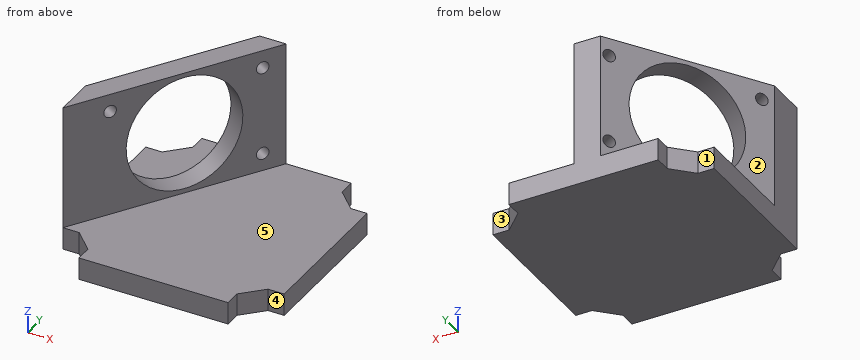
Autodesk Inventor part; units mm, degrees
ref_plane "Work Plane1" through (0, 0, 10) normal (0, 0, 1) x (1, 0, 0)
ref_plane "Work Plane3" through (3.9701, 45.8299, 26) normal (1, 0, 0) x (0, -1, 0)
ref_plane "Work Plane4" through (-34.8055, 8.3289, 16.6138) normal (0.7071, -0.7071, 0) x (0.7071, 0.7071, 0)
ref_plane "Work Plane1" through (0, 0, 10) normal (0, 0, 1) x (1, 0, 0)
sketch "Sketch1" plane through (0, 0, 10) normal (0, 0, 1) x (1, 0, 0)
  line L0 (-4.0299, -0.3538) -> (-2.2322, 1.4439) construction
  arc A0 (-1.4439, 2.2322) -> (-2.2322, 1.4439) centre (-0.9299, 0.9299) ccw construction
  line L1 (-1.4439, 2.2322) -> (0.3538, 4.0299) construction
  line L2 (-37.8299, 42.8299) -> (-37.8299, 37.8299) construction
  line L3 (-37.8299, 37.8299) -> (-42.9208, 37.8299) construction
  line L4 (-37.8299, 42.2137) -> (-37.8299, 45.8299) construction
  line L5 (-37.8299, 45.8299) -> (-4.0299, 45.8299) construction
  line L6 (-4.0299, 45.8299) -> (-4.0299, 42.2137) construction
  line L7 (-4.0299, 4.0299) -> (0.3538, 4.0299)
  circle A1 centre (-20.9299, 20.9299) radius 17.5
  line L8 (-20.9299, 58.9723) -> (17.1124, 20.9299) construction
  line L9 (17.1124, 20.9299) -> (-20.9299, -17.1124) construction
  line L10 (-20.9299, -17.1124) -> (-58.9723, 20.9299) construction
  line L11 (-58.9723, 20.9299) -> (-20.9299, 58.9723) construction
  line L12 (-20.9299, 58.9723) -> (-20.9299, -17.1124) construction
  line L13 (17.1124, 20.9299) -> (-58.9723, 20.9299) construction
  line L14 (-20.9299, 58.9723) -> (32.8701, 58.9723) construction
  line L15 (-43.4299, 43.4299) -> (1.5701, 43.4299) construction
  line L16 (1.5701, 43.4299) -> (1.5701, -1.5701) construction
  line L17 (1.5701, -1.5701) -> (-43.4299, -1.5701) construction
  line L18 (-43.4299, -1.5701) -> (-43.4299, 43.4299) construction
  line L19 (-43.4299, 43.4299) -> (1.5701, -1.5701) construction
  line L20 (1.5701, 43.4299) -> (-43.4299, -1.5701) construction
  line L21 (-43.4299, 5.3876) -> (-43.4299, 36.4723)
  line L22 (-43.4299, 36.4723) -> (-36.4723, 43.4299)
  line L23 (-36.4723, 43.4299) -> (-5.3876, 43.4299)
  line L24 (-5.3876, 43.4299) -> (1.5701, 36.4723)
  line L25 (1.5701, 36.4723) -> (1.5701, 5.3876)
  line L26 (1.5701, 5.3876) -> (-5.3876, -1.5701)
  line L27 (-5.3876, -1.5701) -> (-36.4723, -1.5701)
  line L28 (-36.4723, -1.5701) -> (-43.4299, 5.3876)
  line L29 (-4.0299, 42.2137) -> (-37.8299, 42.2137)
  line L30 (-4.0299, -0.3538) -> (-4.0299, 4.0299)
  circle A2 centre (-20.9299, 20.9299) radius 1.4
  line L31 (-10.9299, 10.9299) -> (-30.9299, 10.9299) construction
  line L32 (-30.9299, 10.9299) -> (-30.9299, 30.9299) construction
  line L33 (-30.9299, 30.9299) -> (-10.9299, 30.9299) construction
  line L34 (-10.9299, 30.9299) -> (-10.9299, 10.9299) construction
  line L35 (-10.9299, 10.9299) -> (-30.9299, 30.9299) construction
  line L36 (-30.9299, 10.9299) -> (-10.9299, 30.9299) construction
  circle A3 centre (-30.9299, 30.9299) radius 1.4
  circle A4 centre (-30.9299, 10.9299) radius 1.4
  circle A5 centre (-10.9299, 10.9299) radius 1.4
  line L37 (-45.8299, 37.8299) -> (-42.0723, 37.8299) construction
  line L38 (-42.1723, 37.7299) -> (-45.8299, 37.7299)
  line L39 (-45.8299, 37.7299) -> (-45.8299, 4.1299)
  line L40 (-45.8299, 4.1299) -> (-42.1723, 4.1299)
  line L41 (-42.1723, 4.1299) -> (-42.1723, 37.7299)
  line L42 (-45.8299, 4.0299) -> (-42.0723, 4.0299) construction
  line L43 (-45.8299, 37.8299) -> (-42.0723, 37.8299)
  line L44 (-37.7299, 45.8299) -> (-4.1299, 45.8299)
  line L45 (-4.1299, 45.8299) -> (-4.1299, 42.1723)
  line L46 (-4.1299, 42.1723) -> (-37.7299, 42.1723)
  line L47 (-37.7299, 42.1723) -> (-37.7299, 45.8299)
  line L48 (0.4701, 37.8299) -> (0.4701, 4.0299) construction
  line L49 (0.4701, 4.0299) -> (3.9701, 4.0299) construction
  line L50 (3.9701, 37.8299) -> (3.9701, 4.0299) construction
  line L51 (0.4701, 37.8299) -> (3.9701, 37.8299) construction
  line L52 (-45.8299, -3.9701) -> (-4.0299, -3.9701) construction
  line L53 (0.3124, 37.7299) -> (3.9701, 37.7299)
  line L54 (3.9701, 37.7299) -> (3.9701, 4.1299)
  line L55 (3.9701, 4.1299) -> (0.3124, 4.1299)
  line L56 (0.3124, 4.1299) -> (0.3124, 37.7299)
  line L57 (-4.1713, -0.3538) -> (-37.7299, -0.3538)
  line L58 (-37.7299, -0.3538) -> (-37.7299, -3.9701)
  line L59 (-37.7299, -3.9701) -> (-4.1713, -3.9701)
  line L60 (-4.1713, -3.9701) -> (-4.1713, -0.3538)
  point P0 (-37.8299, 4.0299)
  dimension "d18" = 53.8
  dimension "d19" = 45
  dimension "d20" = 53.8
  dimension "d21" = 45
  dimension "d22" = 45
  dimension "d30" = 20
  dimension "d31" = 20
  dimension "d32" = 2.8
  dimension "d33" = 2.8
  dimension "d34" = 2.8
  dimension "d35" = 2.8
  dimension "d36" = 0.1
  dimension "d37" = 0.1
  dimension "d38" = 0.1
  dimension "d39" = 0.1
extrude "Extrusion1" add sketch "Sketch1" along normal blind 5 contours L30 L26 L57 L28 L41 L22 L46 L24 L56 L7 | L7 L26 L30 | L56 L24 L25 L26 | L26 L25 L24 L53 L54 L55 | L60 L59 L58 L57 L28 L27 L26 | L26 L27 L28 L57 | L46 L22 L29 L24 | L24 L29 L45 | L40 L39 L38 L22 L21 L28 | L28 L21 L22 L41 | L29 L22 L23 L24 | L24 L23 L22 L29 L47 L44 L45 | L47 L29 L22 | A1 | A2 | A3 | A4 | A5
sketch "Sketch4" plane through (0, 0, 15) normal (0, 0, 1) x (1, 0, 0)
  line L0 (-37.7299, 42.1723) -> (-42.1723, 37.7299)
  line L1 (-42.1723, 37.7299) -> (-45.8299, 37.7299)
  line L2 (-45.8299, 37.7299) -> (-45.8299, 4.1299)
  line L3 (-45.8299, 4.1299) -> (-42.1723, 4.1299)
  line L4 (-42.1723, 4.1299) -> (-37.6885, -0.3538)
  line L5 (-37.6885, -0.3538) -> (-37.7299, -0.3538)
  line L6 (-37.7299, -0.3538) -> (-37.7299, -3.9701)
  line L7 (-37.7299, -3.9701) -> (-4.1713, -3.9701)
  line L8 (-4.1713, -3.9701) -> (-4.1713, -0.3538)
  line L9 (-4.1713, -0.3538) -> (0.3124, 4.1299)
  line L10 (0.3124, 4.1299) -> (3.9701, 4.1299)
  line L11 (3.9701, 4.1299) -> (3.9701, 37.7299)
  line L12 (3.9701, 37.7299) -> (0.3124, 37.7299)
  line L13 (0.3124, 37.7299) -> (-4.1299, 42.1723)
  line L14 (-4.1299, 42.1723) -> (-4.1299, 45.8299)
  line L15 (-4.1299, 45.8299) -> (-37.7299, 45.8299)
  line L16 (-37.7299, 45.8299) -> (-37.7299, 42.1723)
  line L17 (-45.8299, 37.7299) -> (-45.8299, 4.1299)
  line L18 (-45.8299, 4.1299) -> (-18.7496, 45.8299)
  line L19 (-45.8299, 4.1299) -> (3.8916, 4.1299) construction
  line L20 (-18.7496, 45.8299) -> (-24.7114, 45.8299)
  line L21 (-4.1299, 45.8299) -> (-37.7299, 45.8299)
  line L22 (-24.7114, 45.8299) -> (-45.8299, 13.3103)
  line L23 (-45.8299, 4.1299) -> (-45.8299, 13.3103)
  circle A0 centre (-40.9299, 0.9299) radius 1.1933
  circle A1 centre (-0.9299, 40.9299) radius 1.4
  line L24 (-40.9299, 0.9299) -> (-0.9299, 40.9299)
  line L25 (0.3124, 37.7299) -> (-4.1299, 42.1723)
  point P0 (0, 0)
  dimension "d40" = 57
  dimension "d59" = 5
extrude "Extrusion4" add sketch "Sketch4" along normal blind 28 contours L15 L18 L2 L22
sketch "Sketch5" plane through (-45.8299, 13.3103, 15) normal (-0.8387, 0.5446, 0) x (-0.5446, -0.8387, 0)
  line L0 (0, 0) -> (-38.7752, 0)
  line L1 (0, 0) -> (0, 28)
  line L2 (-38.7752, 28) -> (0, 28)
  line L3 (-38.7752, 0) -> (-38.7752, 28)
  circle A0 centre (-19.3876, 8.6124) radius 19.3876
  line L4 (-2.8127, 24) -> (-36.8127, 24) construction
  line L5 (-36.8127, 24) -> (-36.8127, 4) construction
  line L6 (-36.8127, 4) -> (-2.8127, 4) construction
  line L7 (-2.8127, 4) -> (-2.8127, 24) construction
  line L8 (-2.8127, 24) -> (-36.8127, 4) construction
  line L9 (-36.8127, 24) -> (-2.8127, 4) construction
  point P0 (-13.7978, -15)
  point P1 (-19.8127, 14)
  dimension "d44" = 34
  dimension "d45" = 20
hole "Hole1" at (-25.7803, 44.1841, 39) at (-25.7803, 44.1841, 19) at (-44.298, 15.6693, 39) at (-35.0391, 29.9267, 29) direction (0.8387, -0.5446, 0) diameter 2.8 depth 12
ref_plane "Work Plane3" through (3.9701, 45.8299, 26) normal (1, 0, 0) x (0, -1, 0)
ref_plane "Work Plane4" through (-34.8055, 8.3289, 16.6138) normal (0.7071, -0.7071, 0) x (0.7071, 0.7071, 0)
sketch "Sketch9" plane through (-45.8299, 13.3103, 15) normal (-0.8387, 0.5446, 0) x (0, 0, 1)
  line L0 (28, 38.7752) -> (28, 0)
  line L1 (0, 17.4316) -> (0, 19.4237)
  line L2 (28, 19.3876) -> (0, 19.3876) construction
  line L3 (0, 0) -> (0, 38.7752)
  line L4 (0, 0) -> (28, 0)
  line L5 (0, 38.7752) -> (28, 38.7752)
  line L6 (14, 38.7752) -> (14, 0) construction
  circle A0 centre (14, 19.3876) radius 13
  point P0 (-15, 13.7978)
  dimension "d60" = 26
extrude "Extrusion7" cut sketch "Sketch9" against normal up to surface (5 mm away) contours A0
properties part number "20_POL_cube_insert_Brewster_Angle_Kinematic_Mount_base_57_degrees"
Check sheet for the modelled part. Datum: model origin and axes. Units: mm. Face numbers are marked on the shaded views. A direction names the side the tool comes from. Give positions to 0.01 mm unless a question says otherwise; leave off trailing zeros. Order: outer loops, then holes, each group sorted by start corner. A loop starts at its lowest first (then second) coordinate and runs counter-clockwise, first axis right, second up. Notation, with made-up numbers: M 27,-33 L 84,-33 A18 cw 84,-17 Z; hole C 0.5,67.25 d3. An arc over 180 degrees is marked long. Answer in a Markdown table with one row per item. Add a question column.
Q1. Sectioned sample at B-B, the plane z = 39.5. Record the boundary of the cut face in (x, y), and give its area (3 significant figures).
Q2. Access from +Z, -Z, +X, -X, +Y, -Y to the whole of each face (thin tool, end or side, straight path). Record for the marked faces 1, 2, 3, 4 and 5.
Q3. Sectioned sample at D-D, the plane z = 18.5. Record the boundary of the cut face in (x, y).
Q4. Gauge pin test, flat ends, axial feed: pin 1 Ø1.1 at (x, z) = (2.5, 11.5) entering from +Y; pin 2 Ø2 at (x, z) = (-23.5, 36.5) entering from -Y; pin 3 Ø1.1 at (y, z) = (44, 13.5) entering from +X. Record the tip position at first contact, or that the pin passes through.
Q5. Sectioned sample at A-A, the plane z = 31. Record the boundary of the cut face in (x, y), and give its area (3 significant figures).
Q6. Thickness scan on L1, parallel to Z at x = -1.5, y = 25; L2, parallel to X at y = 35, z = 15.5; L3, parallel to Y at x = -24.5, z = 41.5. Record the ranges inside material, lowest first.
Q7. Sectioned sample at C-C, the plane x = -5. Record the boundary of the cut face in (y, z), and give its area (3 significant figures).
Verdict:
| question | item | result |
|---|---|---|
| 1 | outline | M -45.83,4.13 L -40.82,11.85 L -45.01,14.57 L -45.83,13.31 Z; M -43.59,16.77 L -39.39,14.04 L -35.25,20.42 L -39.45,23.14 Z; M -31.1,36 L -26.9,33.28 L -22.3,40.36 L -26.49,43.09 Z; M -25.07,45.28 L -20.87,42.56 L -18.75,45.83 L -24.71,45.83 Z |
| 1 | area | 118 mm² |
| 2 | face 1 | +Z, -Z, -X, +Y |
| 2 | face 2 | +Z, -X, +Y |
| 2 | face 3 | +Z, -Z, +X, +Y |
| 2 | face 4 | +Z, -Z, +X, -Y |
| 2 | face 5 | +Z, +X, -Y |
| 3 | outline | M -45.83,4.13 L -35.25,20.42 L -39.45,23.14 L -45.83,13.31 Z; M -31.1,36 L -26.9,33.28 L -22.3,40.36 L -26.49,43.09 Z; M -25.07,45.28 L -20.87,42.56 L -18.75,45.83 L -24.71,45.83 Z |
| 4 | pin 1 | y = 37.73 |
| 4 | pin 2 | y = 36.98 |
| 4 | pin 3 | x = -4.13 |
| 5 | outline | M -45.83,4.13 L -38.07,16.07 L -42.27,18.8 L -45.83,13.31 Z; M -28.27,40.34 L -24.08,37.62 L -18.75,45.83 L -24.71,45.83 Z |
| 5 | area | 92.8 mm² |
| 6 | L1 | 10 to 15 |
| 6 | L2 | -31.74 to -25.78 |
| 6 | L3 | 36.98 to 45.83 |
| 7 | outline | M -3.97,10 L 45.83,10 L 45.83,15 L -3.97,15 Z |
| 7 | area | 249 mm² |
